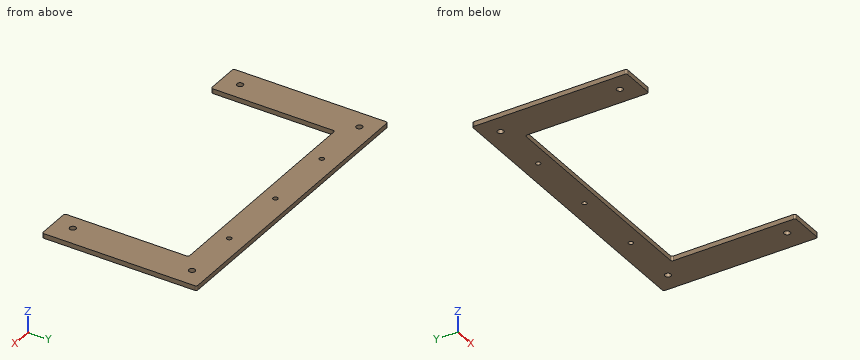
```python
from build123d import *

# Parameters (mm, degrees)
F1_DEPTH = 6.35
F2_R     = 2.54
F3_R     = 4.1656
F4_DEPTH = 25.4
F5_R     = 3.175
F6_DEPTH = 25.4


with BuildPart() as f1:
    # F0 (on Top) → F1 (new body)
    with BuildSketch(Plane.XY):
        Polygon((203.2, 0), (-203.2, 0), (-203.2, -208.28), (-155.575, -208.28), (-155.575, -41.148), (155.575, -41.148), (155.575, -208.28), (203.2, -208.28), align=None)
    extrude(amount=F1_DEPTH)

    # F2
    f2_edges = [f1.edges().sort_by_distance(p)[0] for p in [
        (-155.575, -41.148, 3.175),
        (155.575, -41.148, 3.175),
        (155.575, -208.28, 3.175),
        (-155.575, -208.28, 3.175),
        (-203.2, -208.28, 3.175),
        (203.2, -208.28, 3.175),
        (203.2, 0, 3.175),
        (-203.2, 0, 3.175),
    ]]
    fillet(f2_edges, radius=F2_R)

    # F3 (on face) → F4 (cut)
    with BuildSketch(Plane.XY.offset(6.35)):
        with Locations((-177.693859, -22.225)):
            Circle(F3_R)
        with Locations((-179.604545, -184.15)):
            Circle(F3_R)
        with Locations((177.906141, -22.225)):
            Circle(F3_R)
        with Locations((175.995455, -184.15)):
            Circle(F3_R)
    extrude(amount=-F4_DEPTH, mode=Mode.SUBTRACT)

    # F5 (on face) → F6 (cut)
    with BuildSketch(Plane.XY.offset(6.35)):
        with Locations((0, -22.606)):
            Circle(F5_R)
        with Locations((-98.425, -22.606)):
            Circle(F5_R)
        with Locations((98.425, -22.606)):
            Circle(F5_R)
    extrude(amount=-F6_DEPTH, mode=Mode.SUBTRACT)


solid = f1.part
```
CAD build for the part. Positions are in the model's coordinates, mm. Round coordinates to 2 decimals unless told otherwise and drop trailing zeros. Order: outer loops, then holes, each group sorted by start corner. A loop starts at its lowest first (then second) coordinate and runs counter-clockwise, first axis right, second up.
Q1. Slice it at A-A (y = -164). Write the cut outline in (x, z) (3 decimals), and give its area (3 significant figures).
Q2. Drop a flat-ended pin along its axis: pin 1 (1.9 mm diameter, centred on x = -10, z = 3, fed in from -Y). Give the stop position or say it passes through.
Q3. Slice it at C-C (x = 50.5). Write the cut outline in (y, z), and give its area (3 significant figures).
Q4. Wall check: L1, parallel to X at y = -183.5, z = 5.75 (3 decimals); L2, parallel to X at y = -102.5, z = 5.25 (3 decimals); L3, parallel to Y at x = 0, z = 4.25. Give the ranges that are in metal, low to high.
Q5. Slice it at B-B (z = 1.25). Write the cut outline in (x, y) (3 decimals), and give its area (3 significant figures).
Results below:
1. outline: (-203.2, 0) - (-155.575, 0) - (-155.575, 6.35) - (-203.2, 6.35) - close; (155.575, 0) - (203.2, 0) - (203.2, 6.35) - (155.575, 6.35) - close
1. area: 605 mm2
2. pin 1: stops at y = -41.15
3. outline: (-41.15, 0) - (0, 0) - (0, 6.35) - (-41.15, 6.35) - close
3. area: 261 mm2
4. L1: x = -203.2 to -183.719, -175.49 to -155.575, 155.575 to 171.881, 180.11 to 203.2
4. L2: x = -203.2 to -155.575, 155.575 to 203.2
4. L3: y = -41.15 to -25.78, -19.43 to 0
5. outline: (-203.2, -205.74) arc R2.54 ccw to (-200.66, -208.28) - (-158.115, -208.28) arc R2.54 ccw to (-155.575, -205.74) - (-155.575, -43.688) arc R2.54 cw to (-153.035, -41.148) - (153.035, -41.148) arc R2.54 cw to (155.575, -43.688) - (155.575, -205.74) arc R2.54 ccw to (158.115, -208.28) - (200.66, -208.28) arc R2.54 ccw to (203.2, -205.74) - (203.2, -2.54) arc R2.54 ccw to (200.66, 0) - (-200.66, 0) arc R2.54 ccw to (-203.2, -2.54) - close; hole circle Ø8.331 at (-179.605, -184.15); hole circle Ø8.331 at (-177.694, -22.225); hole circle Ø6.35 at (-98.425, -22.606); hole circle Ø6.35 at (0, -22.606); hole circle Ø6.35 at (98.425, -22.606); hole circle Ø8.331 at (175.995, -184.15); hole circle Ø8.331 at (177.906, -22.225)
5. area: 32,300 mm2
